from build123d import *

# Parameters (mm, degrees)
F0_W          = 187.8567785025
F0_H          = 164.7213101387
F1_DEPTH      = 25.4
F2_DEPTH      = 17.272
F3_R          = 42.1596023767
F3_R_2        = 18.71871866
F4_DEPTH      = 191.262
F4_DEPTH_BACK = 33.782
F5_DEPTH      = 191.263
F7_DEPTH      = 191.263
F7_DEPTH_BACK = 101.6
F8_R          = 16.2084623058
F8_R_2        = 14.6310298949
F9_DEPTH      = 68.073


with BuildPart() as f1:
    # F0 (on Top) → F1 (new body, symmetric)
    with BuildSketch(Plane.XY):
        Rectangle(F0_W, F0_H)
    extrude(amount=F1_DEPTH, both=True)

    # F2 (add, symmetric): a face of the model
    f2_faces = [f1.faces().sort_by_distance(p)[0] for p in [
        (0, 0, 25.4),
    ]]
    extrude(f2_faces, amount=F2_DEPTH, both=True)

    # F3 (on face) → F4 (join, two sides)
    with BuildSketch(Plane.XZ.offset(82.3606550694)) as f4_sk:
        with Locations((0, 42.672)):
            Circle(F3_R)
        with Locations((0, 42.672)):
            Circle(F3_R_2, mode=Mode.SUBTRACT)
    extrude(amount=-F4_DEPTH)
    extrude(f4_sk.sketch, amount=F4_DEPTH_BACK)

    # F3 (on face) → F5 (cut, through all)
    with BuildSketch(Plane.XZ.offset(82.3606550694)):
        with BuildLine():
            ThreePointArc((-18.71871866, 42.672), (0, 23.95328134), (18.71871866, 42.672))
            Line((18.71871866, 42.672), (-18.71871866, 42.672))
        make_face()
    extrude(amount=-F5_DEPTH, mode=Mode.SUBTRACT)

    # F6 (on face) → F7 (cut, two sides)
    with BuildSketch(Plane.XZ.offset(82.3606550694)) as f7_sk:
        Polygon((-50.2506420016, 42.8143106401), (0, 42.8143106401), (50.0124804676, 42.8143106401), (50.0124804676, 85.4440033436), (-50.2506420016, 85.4440033436), align=None)
    extrude(amount=-F7_DEPTH, mode=Mode.SUBTRACT)
    extrude(f7_sk.sketch, amount=F7_DEPTH_BACK, mode=Mode.SUBTRACT)

    # F8 (on face) → F9 (cut, through all)
    with BuildSketch(Plane.XY.offset(42.672)):
        with Locations((-66.1240369081, 0)):
            Circle(F8_R)
        with Locations((65.6378343701, 0)):
            Circle(F8_R_2)
    extrude(amount=-F9_DEPTH, mode=Mode.SUBTRACT)


solid = f1.part
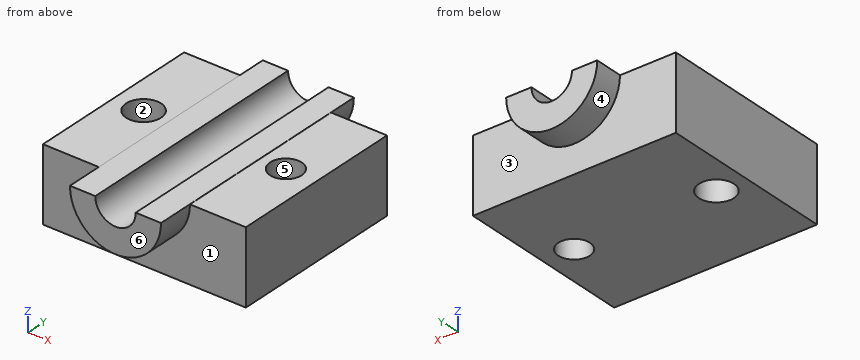
Geometry: final body of the model. Coordinates: model frame, mm. Face numbers are marked on the shaded views. A direction names the side the tool comes from. Give positions to 0.01 mm unless a question says otherwise; leave off trailing zeros. Write each loop counter-clockwise with the first axis right and the second up, starting at its lowest first coordinate (ties: lowest second). Pieces come first, ordered by that corner, then holes. Notation, with made-up numbers: M -34,30 L 16,30 A14 cw 16,51 Z; hole C 37.5,10 d9. An arc over 180 degrees is marked long. Answer in a Markdown table with one row per item. Add a question column.
(1) Mould query, pull axis X, two halves, no side actions, for the marked faces 4, 5 and 6. Classes: +X half, -X half, draft (parallel to the pull), parting line (faces both ways), or undercut.
(2) First-contact query: pin 1 (19.5 mm diameter, centred on x = -66.12, y = 0, fed in from +Z); pin 2 (3 mm diameter, centred on x = -10, y = -38.5, fed in from +Z); pin 3 (2 mm diameter, centred on x = -50, z = 19, fed in from -Y). Flat tips, straight axial feed; report the tip coordinate or a pass-through.
(3) Section D-D on x = 0. Return loops of the section in (y, z).
(4) Section B-B on x = -61. Return loops of the section in (y, z).
(5) Ray query, line 1 (Z direction, x = -54.5, y = -35); line 2 (Y direction, x = -1.5, z = -6); line 3 (X direction, y = 72.5, z = 31.5). Return the intervals inside material, ascending.
(6) Section A-A on y = 0. Return loops of the section in (x, z), and give its area (3 significant figures).
(7) Section C-C on z = 38.5. Return loops of the section in (x, y), and give its area (3 significant figures).
(8) Reachability of the marked faces 1, 2 and 3 from +Z, -Z, +X, -X, +Y, -Y: full face, straight path, thin tool, end or side. Return the list, or none.
Result set:
| question | item | result |
|---|---|---|
| 1 | face 4 | parting line |
| 1 | face 5 | undercut |
| 1 | face 6 | draft |
| 2 | pin 1 | passes through |
| 2 | pin 2 | stops at z = 27.9 |
| 2 | pin 3 | stops at y = -82.36 |
| 3 | outline | M -116.14,0.51 L -82.36,0.51 L -82.36,-25.4 L 82.36,-25.4 L 82.36,0.51 L 108.9,0.51 L 108.9,23.95 L -116.14,23.95 Z |
| 4 | outline | M -82.36,-25.4 L -15.38,-25.4 L -15.38,42.67 L -82.36,42.67 Z; M 15.38,-25.4 L 82.36,-25.4 L 82.36,42.67 L 15.38,42.67 Z |
| 5 | line 1 | z = -25.4 to 42.67 |
| 5 | line 2 | y = -82.36 to 82.36 |
| 5 | line 3 | x = -93.93 to -15.02, 15.02 to 93.93 |
| 6 | outline | M -93.93,-25.4 L -82.33,-25.4 L -82.33,42.67 L -93.93,42.67 Z; M -49.92,-25.4 L 51.01,-25.4 L 51.01,42.67 L 42.16,42.67 A42.16 ccw 42.16,42.81 L 18.72,42.81 A18.72 cw long -18.72,42.81 L -42.16,42.81 A42.16 ccw -42.16,42.67 L -49.92,42.67 Z; M 80.27,-25.4 L 93.93,-25.4 L 93.93,42.67 L 80.27,42.67 Z |
| 6 | area | 8,050 mm^2 |
| 7 | outline | M -93.93,-82.36 L -41.95,-82.36 L -41.95,-116.14 L -18.25,-116.14 L -18.25,108.9 L -41.95,108.9 L -41.95,82.36 L -93.93,82.36 Z; M 18.25,-116.14 L 41.95,-116.14 L 41.95,-82.36 L 93.93,-82.36 L 93.93,82.36 L 41.95,82.36 L 41.95,108.9 L 18.25,108.9 Z; hole C -66.12,0 d32.42; hole C 65.64,0 d29.26 |
| 7 | area | 26,300 mm^2 |
| 8 | face 1 | -Z, -Y |
| 8 | face 2 | +Z, -Z |
| 8 | face 3 | -Z, +Y |
